For this review, take the finished solid that the model builds, in its own axes (mm). Face numbers are marked on the shaded views. Give positions to 0.01 mm unless a question says otherwise; leave off trailing zeros. Order: outer loops, then holes, each group sorted by start corner. A loop starts at its lowest first (then second) coordinate and runs counter-clockwise, first axis right, second up. Notation, with made-up numbers: (77, 60) -> (88, 60) arc R26 ccw to (88, 77) -> close; hole circle Ø2 at (20.25, 54.5). An arc over 180 degrees is marked (long way). Return JSON: item names as keys, results as strings. Group by question number.
1) Add section C-C (y = -4.5). Give the boundary of the cut face in (x, z).
2) The part is to be moulded in two halves that separate along X. For the marked faces 1, 2 and 3, say which applies: released by +X, released by -X, zero draft, split by the parting line, or undercut.
3) To check wall thickness, follow line 1 along Y through (x, z) = (-0.5, 0.85); line 2 along Y through (x, z) = (1.25, 1.4); line 3 along X through (y, z) = (-5, 1.45). State the ranges of each line that lie inside material, in increasing order.
4) Add section A-A (x = 0.25). Give the boundary of the cut face in (y, z).
5) Add section B-B (z = 0.75). Give the boundary of the cut face in (x, y), then the cut area to 3 significant figures.
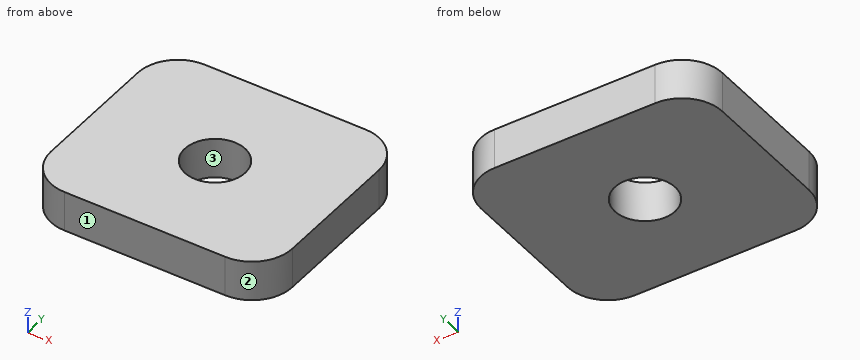
Autodesk Inventor part; units mm, degrees
ref_plane "YZ Plane" through (0, 0, 0) normal (1, 0, 0) x (0, 1, 0)
ref_plane "XZ Plane" through (0, 0, 0) normal (0, 1, 0) x (-1, 0, 0)
ref_plane "XY Plane" through (0, 0, 0) normal (0, 0, 1) x (1, 0, 0)
sketch "washer_sketch" plane through (0, 0, 0) normal (0, 0, 1) x (1, 0, 0)
  line L0 (4.6466, -2.6825) -> (1.9799, -4.6825) construction
  arc A0 (4.6466, -2.6825) -> (5.4466, -1.0825) centre (3.4466, -1.0825) ccw construction
  line L1 (5.4466, 5.0715) -> (5.4466, -1.0825) construction
  line L2 (5.4466, 5.0825) -> (5.4466, 5.0715) construction
  line L3 (-5.4466, 5.0825) -> (5.4466, 5.0825) construction
  line L4 (-5.4466, 0.6191) -> (-5.4466, 5.0825) construction
  arc A1 (-5.4466, 0.6191) -> (-5.0083, -0.6303) centre (-3.4466, 0.6191) ccw construction
  line L5 (-2.0471, -4.3319) -> (-5.0083, -0.6303) construction
  arc A2 (-2.0471, -4.3319) -> (-0.4853, -5.0825) centre (-0.4853, -3.0825) ccw construction
  line L6 (0.7799, -5.0825) -> (-0.4853, -5.0825) construction
  arc A3 (0.7799, -5.0825) -> (1.9799, -4.6825) centre (0.7799, -3.0825) ccw construction
  circle A4 centre (0.0413, -0.1642) radius 3.55 construction
  circle A5 centre (0.0413, -0.1642) radius 3.55 construction
  circle A6 centre (0.0413, -0.1642) radius 1.5
  line L7 (-3.9587, -5.4) -> (4.0413, -5.4)
  line L8 (6.0413, -3.4) -> (6.0413, 3.0715)
  line L9 (4.0413, 5.0715) -> (-3.9587, 5.0715)
  line L10 (-5.9587, 3.0715) -> (-5.9587, -3.4)
  arc A7 (-5.9587, -3.4) -> (-3.9587, -5.4) centre (-3.9587, -3.4) ccw
  arc A8 (-3.9587, 5.0715) -> (-5.9587, 3.0715) centre (-3.9587, 3.0715) ccw
  arc A9 (6.0413, 3.0715) -> (4.0413, 5.0715) centre (4.0413, 3.0715) ccw
  arc A10 (4.0413, -5.4) -> (6.0413, -3.4) centre (4.0413, -3.4) ccw
  point P0 (0, 0)
  point P1 (-5.9587, -5.4)
  point P2 (6.0413, 5.0715)
  point P3 (6.0413, -5.4)
  point P4 (-5.9587, 5.0715)
  dimension "d0" = 10.4715
  dimension "d1" = 12
  dimension "d2" = 5.2358
  dimension "d3" = 6
  dimension "d4" = 2
extrude "washer" add sketch "washer_sketch" along normal blind 2
equation "\"d3\" = 0.5 * d1"
properties part number "mount_linear_stepper_washer_c"
Evaluation:
{
 "1": {"outline": "(-5.63, 0) -> (5.71, 0) -> (5.71, 2) -> (-5.63, 2) -> close"},
 "2": {"face 1": "zero draft", "face 2": "released by +X", "face 3": "undercut"},
 "3": {"line 1": "-5.4 to -1.56, 1.23 to 5.07", "line 2": "-5.4 to -1.05, 0.72 to 5.07", "line 3": "-5.16 to 5.24"},
 "4": {"outline": "(-5.4, 0) -> (-1.65, 0) -> (-1.65, 2) -> (-5.4, 2) -> close; (1.32, 0) -> (5.07, 0) -> (5.07, 2) -> (1.32, 2) -> close"},
 "5": {"outline": "(-5.96, -3.4) arc R2 ccw to (-3.96, -5.4) -> (4.04, -5.4) arc R2 ccw to (6.04, -3.4) -> (6.04, 3.07) arc R2 ccw to (4.04, 5.07) -> (-3.96, 5.07) arc R2 ccw to (-5.96, 3.07) -> close; hole circle Ø3 at (0.04, -0.16)", "area": "115 mm^2"}
}
